For this review, take the finished solid that the model builds, in its own axes (mm). A direction names the side the tool comes from. Coordinates: 2 decimals unless noted, no trailing zeros. Order: outer loops, then holes, each group sorted by start corner. A loop starts at its lowest first (then second) coordinate and runs counter-clockwise, first axis right, second up. Notation, with made-up numbers: (-39.75, -0.75) -> (9.25, -0.75) arc R7 cw to (9.25, 11.25) -> close; hole circle Ø2 at (-13, 51). An arc over 180 degrees is marked (long way). Return JSON: item names as keys, results as strings. Group by question number.
Item 1: Take a section at C-C (z = 4.75). Write out the cut boundary in (x, y).
Item 2: Take a section at A-A (y = 19.75). Write out the cut boundary in (x, z), then the cut area to 3 significant figures.
Item 3: Take a section at B-B (x = 5.2). Write out the cut boundary in (y, z).
Item 4: Draft analysis for pull direction X (two halves, no side actions). For faces 3 (the flat face through (15, 11, 8)), 4 (the cylindrical face through (6.68, 1.64, 7.79)), 5 (the flat face through (7, 11, 15.8)), state which applies: +X half, -X half, draft (parallel to the pull), parting line (faces both ways), or undercut.
Item 5: For line 1 along Y through (x, z) = (5.2, 12); line 2 along Y through (x, z) = (14.5, 13.95); line 3 along X through (y, z) = (2, 12.25), list the stretches that pass through material, from the lowest coordinate up.
Item 6: Insertion check: pin 1 (2 mm diameter, centred on x = 14, y = 11.5, fed in from +Z); pin 2 (3 mm diameter, centred on x = 5.2, y = 19.75, fed in from -Z). Each pin has a flat end and moves straight along its axis. Give the tip position at first contact, or say it passes through.
Item 7: Take a section at D-D (x = 14.5). Write out the cut boundary in (y, z).
Item 8: Machinability: for faces 1 (the flat face through (7, 22, 8)), 2 (the cylindrical face through (12.25, 11.06, 14.32)), which of the approach directions +Z, -Z, +X, -X, +Y, -Y give a long, thin tool a straight path to every point of the face, cutting with its end or side? Answer none if there is none.
```python
from build123d import *

# Parameters (mm, degrees)
SKETCH_1_W          = 15
SKETCH_1_H          = 22
SKETCH_1_R          = 1.6
EXTRUDE_1_DEPTH     = 15.8
SKETCH_2_R          = 2.25
CUT_EXTRUDE_1_DEPTH = 3


with BuildPart() as part:
    # Эскиз1 → Бобышка-Вытянуть1 (new body)
    with BuildSketch(Plane.XY):
        with Locations((7.5, 11)):
            Rectangle(SKETCH_1_W, SKETCH_1_H)
        with Locations((5.2, 19.75)):
            Circle(SKETCH_1_R, mode=Mode.SUBTRACT)
        with Locations((5.2, 2.25)):
            Circle(SKETCH_1_R, mode=Mode.SUBTRACT)
    extrude(amount=EXTRUDE_1_DEPTH)

    # Эскиз2 → Вырез-Вытянуть1 (cut)
    with BuildSketch(Plane.XY.offset(15.8)):
        with Locations((14.5, 11)):
            Circle(SKETCH_2_R)
    extrude(amount=-CUT_EXTRUDE_1_DEPTH, mode=Mode.SUBTRACT)


solid = part.part
```
Findings below:
{
 "1": {"outline": "(0, 0) -> (15, 0) -> (15, 22) -> (0, 22) -> close; hole circle Ø3.2 at (5.2, 2.25); hole circle Ø3.2 at (5.2, 19.75)"},
 "2": {"outline": "(0, 0) -> (3.6, 0) -> (3.6, 15.8) -> (0, 15.8) -> close; (6.8, 0) -> (15, 0) -> (15, 15.8) -> (6.8, 15.8) -> close", "area": "186 mm2"},
 "3": {"outline": "(0, 0) -> (0.65, 0) -> (0.65, 15.8) -> (0, 15.8) -> close; (3.85, 0) -> (18.15, 0) -> (18.15, 15.8) -> (3.85, 15.8) -> close; (21.35, 0) -> (22, 0) -> (22, 15.8) -> (21.35, 15.8) -> close"},
 "4": {"face 3": "+X half", "face 4": "undercut", "face 5": "draft"},
 "5": {"line 1": "y = 0 to 0.65, 3.85 to 18.15, 21.35 to 22", "line 2": "y = 0 to 8.75, 13.25 to 22", "line 3": "x = 0 to 3.62, 6.78 to 15"},
 "6": {"pin 1": "stops at z = 12.8", "pin 2": "passes through"},
 "7": {"outline": "(0, 0) -> (22, 0) -> (22, 15.8) -> (13.25, 15.8) -> (13.25, 12.8) -> (8.75, 12.8) -> (8.75, 15.8) -> (0, 15.8) -> close"},
 "8": {"face 1": "+Z, -Z, +X, -X, +Y", "face 2": "+Z"}
}
